Design review of the part built by this model. Coordinates are the model's own, in mm. Coordinates: 2 decimals unless noted, no trailing zeros. Write each loop counter-clockwise with the first axis right and the second up, starting at its lowest first coordinate (ties: lowest second). Pieces come first, ordered by that corner, then holes. Notation, with made-up numbers: (63.5, 39) - (93.5, 39) arc R16 cw to (93.5, 50) - close; hole circle Ø1 at (11.25, -3.75). An arc over 180 degrees is marked (long way). One line per item, written item: value.
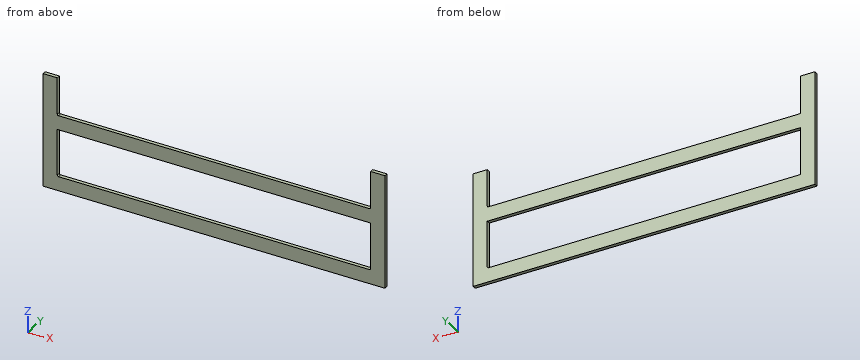
from build123d import *

# Parameters (mm, degrees)
F0_W     = 838.2
F0_H     = 127
F1_DEPTH = 9.525
F2_R     = 3.175


with BuildPart() as f1:
    # F0 (on Front) → F1 (new body)
    with BuildSketch(Plane.XZ):
        Polygon((-487.343022, -18.861064), (-525.443022, -18.861064), (-525.443022, -323.661064), (388.956978, -323.661064), (388.956978, -18.861064), (350.856978, -18.861064), (350.856978, -120.461064), (-487.343022, -120.461064), align=None)
        with Locations((-68.243022, -222.061064)):
            Rectangle(F0_W, F0_H, mode=Mode.SUBTRACT)
    extrude(amount=F1_DEPTH)

    # F2
    f2_edges = [f1.edges().sort_by_distance(p)[0] for p in [
        (-487.343022, -4.7625, -285.561064),
        (350.856978, -4.7625, -285.561064),
        (350.856978, -4.7625, -120.461064),
        (-487.343022, -4.7625, -120.461064),
    ]]
    fillet(f2_edges, radius=F2_R)


solid = f1.part
1. Wall thickness on line 1 along X through (y, z) = (-8, -55.5); line 2 along Z through (x, y) = (285, -2.25): over which ranges is each line inside the solid? List them lowest first.
Answer block:
line 1: x = -525.44 to -487.34, 350.86 to 388.96
line 2: z = -323.66 to -285.56, -158.56 to -120.46
2. Consider section B-B, the plane z = -39.5. Write out the cut boundary in (x, y) (3 decimals), then the cut area to 3 significant figures.
Answer block:
outline: (-525.443, -9.525) - (-487.343, -9.525) - (-487.343, 0) - (-525.443, 0) - close; (350.857, -9.525) - (388.957, -9.525) - (388.957, 0) - (350.857, 0) - close
area: 726 mm^2
3. Consider section C-C, the plane y = -1.75. Write out the cut boundary in (x, z) (3 decimals).
Answer block:
outline: (-525.443, -323.661) - (388.957, -323.661) - (388.957, -18.861) - (350.857, -18.861) - (350.857, -117.286) arc R3.175 cw to (347.682, -120.461) - (-484.168, -120.461) arc R3.175 cw to (-487.343, -117.286) - (-487.343, -18.861) - (-525.443, -18.861) - close; hole (-487.343, -282.386) arc R3.175 ccw to (-484.168, -285.561) - (347.682, -285.561) arc R3.175 ccw to (350.857, -282.386) - (350.857, -158.561) - (-487.343, -158.561) - close
4. Consider section A-A, the plane x = 43.5. Write out the cut boundary in (y, z) (3 decimals).
Answer block:
outline: (-9.525, -323.661) - (0, -323.661) - (0, -285.561) - (-9.525, -285.561) - close; (-9.525, -158.561) - (0, -158.561) - (0, -120.461) - (-9.525, -120.461) - close
5. Insertion check: pin 1 Ø3 at (x, y) = (-181.5, -3.5) entering from +Z. The pin has a flat end and moves straight along its axis. Give the tip position at first contact, or say it passes through.
Answer block:
pin 1: stops at z = -120.46
